Check sheet for the modelled part. Datum: model origin and axes. Units: mm. A direction names the side the tool comes from. Give positions to 0.01 mm unless a question says otherwise; leave off trailing zeros. Order: outer loops, then holes, each group sorted by start corner. A loop starts at its lowest first (then second) coordinate and runs counter-clockwise, first axis right, second up. Notation, with made-up numbers: (-7, 58.5) -> (11, 58.5) arc R17 cw to (11, 62.5) -> close; hole circle Ø9 at (-11.5, -30.75). An arc over 180 degrees is marked (long way). Answer in a Markdown table with one row per item. Add a question column.
(1) Cross-section at B-B (y = 0). Record the cut outline in (x, z), then the cut area to 3 significant figures.
(2) Set-up check for faces 3 (the face through (30.22, 1.15, 4.23)), 4 (the face through (0, 2.5, 1)): record each of +Z, -Z, +X, -X, +Y, -Y from which the full face is reachable in a straight line by a thin tool's end or side.
(3) Cross-section at A-A (z = 2.5). Record the cut outline in (x, y), then the cut area to 3 significant figures.
(4) Thickness scan on L1, parallel to Y at x = 28, z = 5.5; L2, parallel to Y at x = -28, z = 5; L3, parallel to X at y = 0.7, z = 3. Record the ranges inside material, lowest first. Write a range as [from, to].
(5) Release check for a two-part mould opening along X. For faces 1 (the face through (-28, -1, 7)), 2 (the face through (27.15, 0.04, 3.55)) record: released by +X, released by -X, zero draft, split by the parting line, or undercut.
(6) Go/stop test with flat-tipped pins: pin 1 (1.5 mm diameter, centred on x = 7.5, y = -0.5, fed in from +Z); pin 2 (1.4 mm diameter, centred on x = 28, y = 0, fed in from +Z). Record where each tip stops, or that it passes through.
(7) Cross-section at C-C (x = -18.5). Record the cut outline in (y, z), then the cut area to 3 significant figures.
```python
from build123d import *

# Parameters (mm, degrees)
RESSALTO_EXTRUS_O1_DEPTH = 2
ESBO_O3_R                = 2.5
RESSALTO_EXTRUS_O2_DEPTH = 5
ESBO_O5_R                = 2.5
RESSALTO_EXTRUS_O3_DEPTH = 5
ESBO_O2_R                = 0.5
CORTE_EXTRUS_O1_DEPTH    = 32.392674305
ESBO_O4_R                = 0.85
CORTE_EXTRUS_O2_DEPTH    = 32.392674305


with BuildPart() as part:
    # Esboço1 → Ressalto-extrusão1 (new body)
    with BuildSketch(Plane.XY):
        with BuildLine():
            Line((-28, 2.5), (28, 2.5))
            ThreePointArc((28, 2.5), (30.5, 0), (28, -2.5))
            Line((28, -2.5), (-28, -2.5))
            ThreePointArc((-28, -2.5), (-30.5, 0), (-28, 2.5))
        make_face()
    extrude(amount=RESSALTO_EXTRUS_O1_DEPTH)

    # Esboço3 → Ressalto-extrusão2 (add)
    with BuildSketch(Plane.XY.offset(2)):
        with Locations(Location((28, 0, 0), (0, 0, 90))):
            Circle(ESBO_O3_R)
    extrude(amount=RESSALTO_EXTRUS_O2_DEPTH)

    # Esboço5 → Ressalto-extrusão3 (add)
    with BuildSketch(Plane.XY.offset(2)):
        with Locations(Location((-28, 0, 0), (0, 0, 270))):
            Circle(ESBO_O5_R)
    extrude(amount=RESSALTO_EXTRUS_O3_DEPTH)

    # Esboço2 → Corte-extrusão1 (cut, through all)
    with BuildSketch(Plane.XY.offset(7)):
        with Locations((-28, 0)):
            Circle(ESBO_O2_R)
    extrude(amount=-CORTE_EXTRUS_O1_DEPTH, mode=Mode.SUBTRACT)

    # Esboço4 → Corte-extrusão2 (cut, through all)
    with BuildSketch(Plane.XY.offset(7)):
        with Locations((28, 0)):
            Circle(ESBO_O4_R)
    extrude(amount=-CORTE_EXTRUS_O2_DEPTH, mode=Mode.SUBTRACT)


solid = part.part
```
Answer below:
| question | item | result |
|---|---|---|
| 1 | outline | (-30.5, 0) -> (-28.5, 0) -> (-28.5, 7) -> (-30.5, 7) -> close; (-27.5, 0) -> (27.15, 0) -> (27.15, 7) -> (25.5, 7) -> (25.5, 2) -> (-25.5, 2) -> (-25.5, 7) -> (-27.5, 7) -> close; (28.85, 0) -> (30.5, 0) -> (30.5, 7) -> (28.85, 7) -> close |
| 1 | area | 153 mm² |
| 2 | face 3 | +Z |
| 2 | face 4 | +Z, -Z, +X, -X, +Y |
| 3 | outline | circle Ø5 at (-28, 0); circle Ø5 at (28, 0); hole circle Ø1 at (-28, 0); hole circle Ø1.7 at (28, 0) |
| 3 | area | 36.2 mm² |
| 4 | L1 | y = [-2.5, -0.85], [0.85, 2.5] |
| 4 | L2 | y = [-2.5, -0.5], [0.5, 2.5] |
| 4 | L3 | x = [-30.4, -25.6], [25.6, 27.52], [28.48, 30.4] |
| 5 | face 1 | zero draft |
| 5 | face 2 | undercut |
| 6 | pin 1 | stops at z = 2 |
| 6 | pin 2 | passes through |
| 7 | outline | (-2.5, 0) -> (2.5, 0) -> (2.5, 2) -> (-2.5, 2) -> close |
| 7 | area | 10.0 mm² |
